Work out the finished part from the listing and answer in its coordinate system (mm). A direction names the side the tool comes from. Round coordinates to 2 decimals unless told otherwise and drop trailing zeros. Write each loop counter-clockwise with the first axis right and the second up, starting at its lowest first coordinate (ties: lowest second). Pieces come first, ordered by that corner, then holes. Notation, with made-up numbers: (23.5, 43.25) -> (45.5, 43.25) arc R24 cw to (45.5, 62.25) -> close; hole circle Ø3 at (-34, -38). An arc over 180 degrees is marked (long way). One line per question, with ' | ' between items. Start each with the question number.
```python
from build123d import *

# Parameters (mm, degrees)
SKETCH1_W                            = 38.1
SKETCH1_H                            = 25.4
SKETCH1_W_2                          = 33.3375
SKETCH1_H_2                          = 20.6375
BOSS_EXTRUDE1_DEPTH                  = 127
SKETCH2_R                            = 12.7
CUT_EXTRUDE1_DEPTH                   = 136.002851822
SKETCH3_R                            = 6.35
SKETCH3_R_2                          = 1.778
CUT_EXTRUDE2_DEPTH                   = 136.002851822
CUT_EXTRUDE3_REACH                   = 137.003
F_4_0_209_DIAMETER_HOLE1_D           = 3.556
F_4_0_209_DIAMETER_HOLE1_ON_FACE_2_D = 3.556
F_4_0_209_DIAMETER_HOLE1_ON_FACE_3_D = 3.556
F_4_0_209_DIAMETER_HOLE1_ON_FACE_4_D = 3.556
CUT_EXTRUDE4_REACH                   = 137.003


with BuildPart() as part:
    # Sketch1 → Boss-Extrude1 (new body)
    with BuildSketch(Plane(origin=(0, 0, 0), x_dir=(0, 0, -1), z_dir=(1, 0, 0))):
        with Locations((19.05, 12.7)):
            Rectangle(SKETCH1_W, SKETCH1_H)
        with Locations((19.05, 12.7)):
            Rectangle(SKETCH1_W_2, SKETCH1_H_2, mode=Mode.SUBTRACT)
    extrude(amount=BOSS_EXTRUDE1_DEPTH)

    # Sketch2 → Cut-Extrude1 (cut, through all)
    with BuildSketch(Plane(origin=(0, 25.4, 0), x_dir=(1, 0, 0), z_dir=(0, 1, 0))):
        with Locations(Location((23.495, 19.05, 0), (0, 0, 270))):
            Circle(SKETCH2_R)
    extrude(amount=-CUT_EXTRUDE1_DEPTH, mode=Mode.SUBTRACT)

    # Sketch3 → Cut-Extrude2 (cut, through all)
    with BuildSketch(Plane.XY):
        with Locations((23.495, 12.7)):
            Circle(SKETCH3_R)
        with Locations((16.580202787, 19.614797213)):
            Circle(SKETCH3_R_2)
        with Locations((16.580202787, 5.785202787)):
            Circle(SKETCH3_R_2)
        with Locations((30.409797213, 5.785202787)):
            Circle(SKETCH3_R_2)
        with Locations((30.409797213, 19.614797213)):
            Circle(SKETCH3_R_2)
        with BuildLine():
            Line((46.355, 22.225), (60.325, 22.225))
            ThreePointArc((60.325, 22.225), (62.57006403, 21.29506403), (63.5, 19.05))
            Line((63.5, 19.05), (63.5, 6.35))
            ThreePointArc((63.5, 6.35), (62.57006403, 4.10493597), (60.325, 3.175))
            Line((60.325, 3.175), (46.355, 3.175))
            ThreePointArc((46.355, 3.175), (44.10993597, 4.10493597), (43.18, 6.35))
            Line((43.18, 6.35), (43.18, 19.05))
            ThreePointArc((43.18, 19.05), (44.10993597, 21.29506403), (46.355, 22.225))
        make_face()
        with BuildLine():
            Line((73.025, 22.225), (86.995, 22.225))
            ThreePointArc((86.995, 22.225), (89.24006403, 21.29506403), (90.17, 19.05))
            Line((90.17, 19.05), (90.17, 6.35))
            ThreePointArc((90.17, 6.35), (89.24006403, 4.10493597), (86.995, 3.175))
            Line((86.995, 3.175), (73.025, 3.175))
            ThreePointArc((73.025, 3.175), (70.77993597, 4.10493597), (69.85, 6.35))
            Line((69.85, 6.35), (69.85, 19.05))
            ThreePointArc((69.85, 19.05), (70.77993597, 21.29506403), (73.025, 22.225))
        make_face()
        with BuildLine():
            Line((99.695, 22.225), (113.665, 22.225))
            ThreePointArc((113.665, 22.225), (115.91006403, 21.29506403), (116.84, 19.05))
            Line((116.84, 19.05), (116.84, 6.35))
            ThreePointArc((116.84, 6.35), (115.91006403, 4.10493597), (113.665, 3.175))
            Line((113.665, 3.175), (99.695, 3.175))
            ThreePointArc((99.695, 3.175), (97.44993597, 4.10493597), (96.52, 6.35))
            Line((96.52, 6.35), (96.52, 19.05))
            ThreePointArc((96.52, 19.05), (97.44993597, 21.29506403), (99.695, 22.225))
        make_face()
    extrude(amount=-CUT_EXTRUDE2_DEPTH, mode=Mode.SUBTRACT)

    # Sketch4 → Cut-Extrude3 (cut, up to next)
    with BuildSketch(Plane(origin=(0, 25.4, 0), x_dir=(1, 0, 0), z_dir=(0, 1, 0)), mode=Mode.PRIVATE) as cut_extrude3_sk1:
        with BuildLine():
            Line((43.575463142, 6.35), (113.665, 6.35))
            ThreePointArc((113.665, 6.35), (115.91006403, 7.27993597), (116.84, 9.525))
            Line((116.84, 9.525), (116.84, 32.385))
            ThreePointArc((116.84, 32.385), (115.91006403, 34.63006403), (113.665, 35.56))
            Line((113.665, 35.56), (41.275, 35.56))
            ThreePointArc((41.275, 35.56), (38.435193669, 33.804903166), (38.735, 30.48))
            ThreePointArc((38.735, 30.48), (42.449267423, 20.957418792), (40.70682555, 10.885714286))
            ThreePointArc((40.70682555, 10.885714286), (40.892098383, 7.827891114), (43.575463142, 6.35))
        make_face()
    cut_extrude3_tool1 = extrude(cut_extrude3_sk1.sketch, amount=-CUT_EXTRUDE3_REACH, mode=Mode.PRIVATE) & part.part
    add(cut_extrude3_tool1.solids().sort_by_distance((78.81497, 25.4, -21.04719))[0], mode=Mode.SUBTRACT)

    # #4 (0.209) Diameter Hole1 (through all)
    with Locations(Plane(origin=(3.175, 25.4, -19.05), x_dir=(0, 0, 1), z_dir=(0, 1, 0))):
        with Locations((0, 0), (0, 120.65)):
            Hole(F_4_0_209_DIAMETER_HOLE1_D / 2)

    # #4 (0.209) Diameter Hole1 on face 2 (through all)
    with Locations(Plane(origin=(123.825, 12.7, 0), x_dir=(1, 0, 0), z_dir=(0, 0, 1))):
        with Locations((0, 0), (-120.65, 0)):
            Hole(F_4_0_209_DIAMETER_HOLE1_ON_FACE_2_D / 2)

    # #4 (0.209) Diameter Hole1 on face 3 (through all)
    with Locations(Plane(origin=(123.825, 0, -19.05), x_dir=(0, 0, -1), z_dir=(0, -1, 0))):
        with Locations((0, 0), (0, -120.65)):
            Hole(F_4_0_209_DIAMETER_HOLE1_ON_FACE_3_D / 2)

    # #4 (0.209) Diameter Hole1 on face 4 (through all)
    with Locations(Plane(origin=(123.825, 12.7, -38.1), x_dir=(-1, 0, 0), z_dir=(0, 0, -1))):
        with Locations((0, 0), (120.65, 0)):
            Hole(F_4_0_209_DIAMETER_HOLE1_ON_FACE_4_D / 2)

    # Sketch6 → Cut-Extrude4 (cut, up to next)
    with BuildSketch(Plane.XZ, mode=Mode.PRIVATE) as cut_extrude4_sk1:
        with BuildLine():
            Line((48.26, -35.56), (107.95, -35.56))
            ThreePointArc((107.95, -35.56), (111.125, -32.385), (107.95, -29.21))
            Line((107.95, -29.21), (107.95, -24.13))
            Line((107.95, -24.13), (111.125, -24.13))
            ThreePointArc((111.125, -24.13), (114.3, -20.955), (111.125, -17.78))
            Line((111.125, -17.78), (107.95, -17.78))
            Line((107.95, -17.78), (107.95, -12.7))
            ThreePointArc((107.95, -12.7), (111.125, -9.525), (107.95, -6.35))
            Line((107.95, -6.35), (48.26, -6.35))
            ThreePointArc((48.26, -6.35), (45.085, -9.525), (48.26, -12.7))
            Line((48.26, -12.7), (48.26, -17.78))
            Line((48.26, -17.78), (45.085, -17.78))
            ThreePointArc((45.085, -17.78), (41.91, -20.955), (45.085, -24.13))
            Line((45.085, -24.13), (48.26, -24.13))
            Line((48.26, -24.13), (48.26, -29.21))
            ThreePointArc((48.26, -29.21), (45.085, -32.385), (48.26, -35.56))
        make_face()
    cut_extrude4_tool1 = extrude(cut_extrude4_sk1.sketch, amount=-CUT_EXTRUDE4_REACH, mode=Mode.PRIVATE) & part.part
    add(cut_extrude4_tool1.solids().sort_by_distance((78.105, 0, -20.955))[0], mode=Mode.SUBTRACT)


solid = part.part
```
(1) For faces 1 (the flat face through (47, 1, -17.78)), 2 (the flat face through (78, 24, -6.35)), 3 (the cylindrical face through (97.475, 4.08, -36.893)), determine the directions among +Z, -Z, +X, -X, +Y, -Y from which every point of the face is accessible in a straight line to the end or side of a thin tool.
(2) Consider L1, parallel to X at y = 1.65, z = -19.05 (3 decimals); L2, parallel to Y at x = 34.5, z = -8; L3, parallel to X at y = 23.6, z = -19.05 (3 decimals). Determine where each line is inside the solid, lowest interval first.
(3) A cutting plane is placed at B-B, the plane z = -27. Determine the outline of the cut face in (x, y), then the cut area to 3 significant figures.
(4) A cutting plane is placed at C-C, the plane x = 115.5. Determine the outline of the cut face in (y, z).
(5) The mould has two halves that part along X. Classify faces 4 (the cylindrical face through (70.755, 21.27, -1.174)), 5 (the flat face through (0, 24, -19)), 6 (the flat face through (63, 2.381, -4)): +X half, -X half, draft (parallel to the pull), parting line (faces both ways), or undercut.
(6) A cutting plane is placed at D-D, the plane y = 12.7. Count the separate pieces of the cut face and the enclosed holes in it, then the cut area to 3 significant figures.
(7) A cutting plane is placed at A-A, the plane x = 71. Determine the outline of the cut face in (y, z), then the cut area to 3 significant figures.
(8) Given pin 1 Ø4.5 at (x, y) = (30.41, 19.61) entering from -Z; pin 2 Ø8 at (x, z) = (19, -12.5) entering from -Y, each flat-ended and moving along its own axis, determine where each tip first touches the part or whether it passes through.
Returned:
1) face 1: +Y, -Y | face 2: +Y | face 3: +Z, -Z
2) L1: 0 to 1.397, 4.953 to 10.795, 36.195 to 42.545, 113.665 to 122.047, 125.603 to 127 | L2: 0 to 2.38, 23.02 to 25.4 | L3: 0 to 1.397, 4.953 to 10.795, 36.195 to 42.545, 116.84 to 122.047, 125.603 to 127
3) outline: (0, 0) -> (13.59, 0) -> (13.59, 2.38) -> (0, 2.38) -> close; (0, 23.02) -> (13.59, 23.02) -> (13.59, 25.4) -> (0, 25.4) -> close; (33.4, 0) -> (48.26, 0) -> (48.26, 2.38) -> (33.4, 2.38) -> close; (33.4, 23.02) -> (40.81, 23.02) -> (40.81, 25.4) -> (33.4, 25.4) -> close; (107.95, 0) -> (127, 0) -> (127, 2.38) -> (107.95, 2.38) -> close; (116.84, 23.02) -> (127, 23.02) -> (127, 25.4) -> (116.84, 25.4) -> close | area: 187 mm2
4) outline: (0, -38.1) -> (3.76, -38.1) -> (3.76, -35.72) -> (2.38, -35.72) -> (2.38, -2.38) -> (3.76, -2.38) -> (3.76, 0) -> (0, 0) -> close; (21.64, -38.1) -> (25.4, -38.1) -> (25.4, -34.98) -> (23.02, -34.98) -> (23.02, -35.72) -> (21.64, -35.72) -> close; (21.64, -2.38) -> (23.02, -2.38) -> (23.02, -6.93) -> (25.4, -6.93) -> (25.4, 0) -> (21.64, 0) -> close
5) face 4: undercut | face 5: -X half | face 6: draft
6) separate pieces: 14 | enclosed holes: 0 | area: 220 mm2
7) outline: (0, -38.1) -> (3.9, -38.1) -> (3.9, -35.72) -> (2.38, -35.72) -> (2.38, -35.56) -> (0, -35.56) -> close; (0, -6.35) -> (2.38, -6.35) -> (2.38, -2.38) -> (3.9, -2.38) -> (3.9, 0) -> (0, 0) -> close; (21.5, -38.1) -> (25.4, -38.1) -> (25.4, -35.56) -> (23.02, -35.56) -> (23.02, -35.72) -> (21.5, -35.72) -> close; (21.5, -2.38) -> (23.02, -2.38) -> (23.02, -6.35) -> (25.4, -6.35) -> (25.4, 0) -> (21.5, 0) -> close | area: 56.8 mm2
8) pin 1: z = -38.1 | pin 2: through
